Autodesk Inventor part; units mm, degrees
ref_plane "YZ Plane" through (0, 0, 0) normal (1, 0, 0) x (0, 1, 0)
ref_plane "XZ Plane" through (0, 0, 0) normal (0, 1, 0) x (-1, 0, 0)
ref_plane "XY Plane" through (0, 0, 0) normal (0, 0, 1) x (1, 0, 0)
sketch "Sketch1" plane through (0, 0, 0) normal (0, 1, 0) x (-1, 0, 0)
  line L0 (3.5, 5) -> (-3.5, 5)
  line L1 (-3.5, 5) -> (-3.5, -5)
  line L2 (-3.5, -5) -> (3.5, -5)
  line L3 (3.5, -5) -> (3.5, 5)
  line L4 (3.5, 5) -> (-3.5, -5) construction
  line L5 (-3.5, 5) -> (3.5, -5) construction
  line L6 (-1.5, 5) -> (-3.5, 3.5)
  line L7 (-1.5, -5) -> (-3.5, -3.5)
  line L8 (5.5, 3) -> (1.5, 3)
  line L9 (1.5, 3) -> (1.5, -3)
  line L10 (1.5, -3) -> (5.5, -3)
  line L11 (5.5, -3) -> (5.5, 3)
  line L12 (5.5, 3) -> (1.5, -3) construction
  line L13 (1.5, 3) -> (5.5, -3) construction
  point P0 (0, 0)
  point P1 (-3.5, 0)
  point P2 (3.5, 0)
  point P3 (3.5, 3)
  point P4 (3.5, -3)
  dimension "d0" = 7
  dimension "d1" = 10
  dimension "d2" = 5
  dimension "d3" = 5
  dimension "d4" = 3.5
  dimension "d5" = 3.5
  dimension "d6" = 4
  dimension "d7" = 6
extrude "Extrusion1" add sketch "Sketch1" along normal blind 15 contours L3 L8 L9 L10 L2 L7 L1 L6 L0 | L8 L11 L10 L3 | L3 L10 L9 L8
sketch "Sketch2" plane through (-5.5, 0, -3) normal (-1, 0, 0) x (0, 0, 1)
  circle A0 centre (3, 7.5) radius 2.4
  line L0 (0, 0) -> (6, 0)
  line L1 (0, 0) -> (0, 15)
  point P0 (3, 0)
  dimension "d10" = 4.8
  dimension "d11" = 7.5
  dimension "d12" = 3
extrude "Extrusion2" cut sketch "Sketch2" against normal through all
thread "Thread1"
properties part number "drazka"
Can you work these out from the model? Positions are in its coordinate system, mm. A direction names the side the tool comes from. Coordinates: 2 decimals unless noted, no trailing zeros. Loops run counter-clockwise (first coordinate to the right, second up) from the corner with the lowest first, then second, coordinate; pieces in that order, holes last.
Item 1: Which directions (+Z, -Z, +X, -X, +Y, -Y) give clear straight access to the entire face, cutting with the end or side of a thin tool? Please do faces 4 (the face through (-5, 7, 3)), 5 (the face through (2.49, 7.4, -4.26)), 6 (the face through (-3.5, 7, -4)).
Answers below:
face 4: +Z, -X, +Y, -Y
face 5: -Z, +X, +Y, -Y
face 6: -Z, -X, +Y, -Y
Item 2: Suppose I cut it at A-A (y = 7.5). Please give me the cut outline in (x, z).
Answers below:
outline: (-5.5, -3) - (-3.5, -3) - (-3.5, -5) - (1.5, -5) - (3.5, -3.5) - (3.5, -2.4) - (-5.5, -2.4) - close; (-5.5, 2.4) - (3.5, 2.4) - (3.5, 3.5) - (1.5, 5) - (-3.5, 5) - (-3.5, 3) - (-5.5, 3) - close
Item 3: Suppose I cut it at C-C (x = -4.25). Please give me the cut outline in (y, z).
Answers below:
outline: (0, -3) - (15, -3) - (15, 3) - (0, 3) - close; hole circle Ø4.8 at (7.5, 0)
Item 4: Suppose I cut it at D-D (y = 10.5). Please give me the cut outline in (x, z).
Answers below:
outline: (-5.5, -3) - (-3.5, -3) - (-3.5, -5) - (1.5, -5) - (3.5, -3.5) - (3.5, 3.5) - (1.5, 5) - (-3.5, 5) - (-3.5, 3) - (-5.5, 3) - close
Item 5: Please list where these lines run through material, in increasing order: L1, parallel to Y at x = -0.75, z = 0; L2, parallel to Z at x = -1, y = 6; L3, parallel to Y at x = -0.25, z = -1.25.
Answers below:
L1: y = 0 to 5.1, 9.9 to 15
L2: z = -5 to -1.87, 1.87 to 5
L3: y = 0 to 5.45, 9.55 to 15
Item 6: Suppose I cut it at B-B (z = 0). Please give me the cut outline in (x, y).
Answers below:
outline: (-5.5, 0) - (3.5, 0) - (3.5, 5.1) - (-5.5, 5.1) - close; (-5.5, 9.9) - (3.5, 9.9) - (3.5, 15) - (-5.5, 15) - close
Item 7: If we mould it in two halves opening along Z, with no side actions, what happens to faces 1 (the face through (-1.063, 9.524, 1.29)), 2 (the face through (-1, 7, -5)), 3 (the face through (3.5, 9.1, -2.3))? For each: released by +Z, released by -Z, zero draft, split by the parting line, or undercut.
Answers below:
face 1: undercut
face 2: released by -Z
face 3: zero draft
Item 8: I'm going to push flat-ended pins straight in: pin 1 (1.6 mm diameter, centred on y = 6.5, z = 4.5, fed in from -X); pin 2 (4.5 mm diameter, centred on y = 7.5, z = 0, fed in from -X). Where does each tip first touch, or does it pass through?
Answers below:
pin 1: stops at x = -3.5
pin 2: passes through
